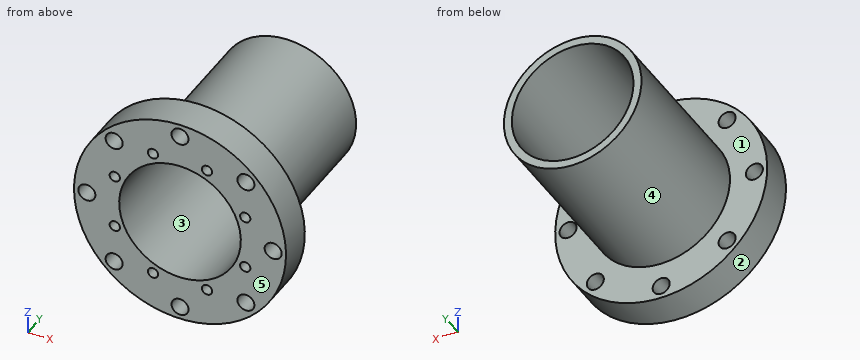
from build123d import *

# Parameters (mm, degrees)
SKETCH1_R               = 34.036
EXTRUDE1_DEPTH          = 82.55
SKETCH2_R               = 52.451
EXTRUDE2_DEPTH          = 17.526
CUT_EXTRUDE1_DEPTH      = 111.980706891
CUT_EXTRUDE1_DEPTH_BACK = 111.980706891
SKETCH3_R               = 30.099
SKETCH4_R               = 4.2164
CUT_EXTRUDE2_DEPTH      = 17.526
CIRPATTERN1_COUNT       = 8
CIRPATTERN3_COUNT       = 8


with BuildPart() as part:
    # Sketch1 → Extrude1 (new body)
    with BuildSketch(Plane(origin=(0, 0, 0), x_dir=(1, 0, 0), z_dir=(0, 1, 0))):
        with Locations(Location((0, 0, 0), (0, 0, 270))):
            Circle(SKETCH1_R)
    extrude(amount=EXTRUDE1_DEPTH)

    # Sketch2 → Extrude2 (add)
    with BuildSketch(Plane(origin=(0, 0, 0), x_dir=(1, 0, 0), z_dir=(0, 1, 0))):
        with Locations(Location((0, 0, 0), (0, 0, 270))):
            Circle(SKETCH2_R)
    extrude(amount=-EXTRUDE2_DEPTH)

    # Sketch3 → Cut-Extrude1 (cut, two sides: drawn at the far end of the back side and taken through both)
    with BuildSketch(Plane(origin=(0, 0, 0), x_dir=(1, 0, 0), z_dir=(0, 1, 0)).offset(-CUT_EXTRUDE1_DEPTH_BACK)):
        with Locations(Location((0, 0, 0), (0, 0, 270))):
            Circle(SKETCH3_R)
    extrude(amount=CUT_EXTRUDE1_DEPTH + CUT_EXTRUDE1_DEPTH_BACK, mode=Mode.SUBTRACT)

    # Sketch4 → Cut-Extrude2 (cut)
    with BuildSketch(Plane(origin=(0, 0, 0), x_dir=(1, 0, 0), z_dir=(0, 1, 0))):
        with Locations(Location((0, 46.101, 0), (0, 0, 270))):
            Circle(SKETCH4_R)
    cut_extrude2 = extrude(amount=-CUT_EXTRUDE2_DEPTH, mode=Mode.SUBTRACT)

    # CirPattern1: Cut-Extrude2 ×8 about axis
    cirpattern1_axis = Axis((0, 0, 0), (0, 1, 0))
    for i in range(1, CIRPATTERN1_COUNT):
        add(cut_extrude2.rotate(cirpattern1_axis, i * 360 / CIRPATTERN1_COUNT), mode=Mode.SUBTRACT)

    # Sketch10 → 1_4-20 Tapped Hole2 (revolve, cut)
    with BuildSketch(Plane(origin=(13.365218875, -17.526, 32.266492673), x_dir=(0, 0, -1), z_dir=(1, 0, 0))):
        Polygon((0, 0), (0, 15.503816902), (2.5527, 13.97), (2.5527, 0), align=None)
    f_1_4_20_tapped_hole2 = revolve(axis=Axis((13.365218875, -23.876, 32.266492673), (0, 1, 0)), mode=Mode.SUBTRACT)

    # CirPattern3: 1_4-20 Tapped Hole2 ×8 about axis
    cirpattern3_axis = Axis((0, 0, 0), (0, 1, 0))
    for i in range(1, CIRPATTERN3_COUNT):
        add(f_1_4_20_tapped_hole2.rotate(cirpattern3_axis, i * 360 / CIRPATTERN3_COUNT), mode=Mode.SUBTRACT)


solid = part.part
Build history of the part. All positions in model axes, mm. Face numbers are marked on the shaded views. A direction names the side the tool comes from. Coordinates: 2 decimals unless noted, no trailing zeros. Order: outer loops, then holes, each group sorted by start corner. A loop starts at its lowest first (then second) coordinate and runs counter-clockwise, first axis right, second up. Notation, with made-up numbers: (10.5, 42.25) - (25.5, 42.25) arc R30 cw to (25.5, 70.25) - close; hole circle Ø9 at (55, 12.5). An arc over 180 degrees is marked (long way). Write item = value, one per line. Start each with the question number.
1) Saw through at C-C on x = 24. Write the cut outline in (y, z).
2) 3-axis set-ups, long thin cutter, end or side, ignore diameter. For the marked faces 4 and 5: which of +Z, -Z, +X, -X, +Y, -Y reach the whole face in a straight line?
3) Flat gauge pins, fed straight in: pin 1 Ø4.5 at (x, z) = (13.37, -32.27) entering from -Y; pin 2 Ø11 at (x, z) = (-46.101, 0) entering from +Y; pin 3 Ø8 at (y, z) = (51, -30) entering from -X. Where does each tip first touch, or does it go through?
4) Saw through at D-D on y = -10.5. Count the separate pieces of the cut face and the enclosed holes in it, then the cut area to 3 significant figures.
5) Saw through at B-B on z = 0. Write the cut outline in (x, y), then the cut area to 3 significant figures.
6) Two-plate mould, pull along Z, no slides. Class the marked faces 1, 2 and 3: pulls with the +Z half, pulls with the -Z half, needs draft (parallel to the pull), parting line crosses it, or undercut.
7) Saw through at A-A on x = 0. Write the cut outline in (y, z).
8) Wall check: line 1 along Z through (x, y) = (11.5, 2); line 2 along X through (y, z) = (75, 15); line 3 along Y through (x, z) = (40, -14). Give the ranges that are in metal, low to high. Write a range as from..to.
From the geometry:
q1.outline = (-17.53, -46.64) - (0, -46.64) - (0, -24.13) - (82.55, -24.13) - (82.55, -18.16) - (-17.53, -18.16) - close; (-17.53, 18.16) - (82.55, 18.16) - (82.55, 24.13) - (0, 24.13) - (0, 46.64) - (-17.53, 46.64) - close
q2.face_4 = +Y
q2.face_5 = +Z, -Z, +X, -X, -Y
q3.pin_1 = -3.38
q3.pin_2 = 0
q3.pin_3 = -21.96
q4.separate_pieces = 1
q4.enclosed_holes = 17
q4.area = 5,190 mm^2
q5.outline = (-52.45, -17.53) - (-50.32, -17.53) - (-50.32, 0) - (-52.45, 0) - close; (-41.88, -17.53) - (-30.1, -17.53) - (-30.1, 82.55) - (-34.04, 82.55) - (-34.04, 0) - (-41.88, 0) - close; (30.1, -17.53) - (41.88, -17.53) - (41.88, 0) - (34.04, 0) - (34.04, 82.55) - (30.1, 82.55) - close; (50.32, -17.53) - (52.45, -17.53) - (52.45, 0) - (50.32, 0) - close
q5.area = 1,140 mm^2
q6.face_1 = needs draft
q6.face_2 = parting line crosses it
q6.face_3 = undercut
q7.outline = (-17.53, -52.45) - (0, -52.45) - (0, -50.32) - (-17.53, -50.32) - close; (-17.53, -41.88) - (0, -41.88) - (0, -34.04) - (82.55, -34.04) - (82.55, -30.1) - (-17.53, -30.1) - close; (-17.53, 30.1) - (82.55, 30.1) - (82.55, 34.04) - (0, 34.04) - (0, 41.88) - (-17.53, 41.88) - close; (-17.53, 50.32) - (0, 50.32) - (0, 52.45) - (-17.53, 52.45) - close
q8.line_1 = -32.03..-27.82, 27.82..32.03
q8.line_2 = -30.55..-26.1, 26.1..30.55
q8.line_3 = -17.53..0
